The model under review builds one solid part; all positions refer to its coordinate system, in mm. A direction names the side the tool comes from. Round coordinates to 2 decimals unless told otherwise and drop trailing zeros. Loops run counter-clockwise (first coordinate to the right, second up) from the corner with the lowest first, then second, coordinate; pieces in that order, holes last. Notation, with made-up numbers: (14, 82) -> (33, 82) arc R34 cw to (33, 120) -> close; hole circle Ø6 at (34.5, -16.5). An arc over 180 degrees is marked (long way). Use a Markdown table: item, result. Add a question column.
1) Consider section A-A on x = 0. Give the boundary of the cut face in (y, z).
2) For faces 1 (the flat face through (-5, -4, 0)), 2 (the flat face through (5, 4, 0)), 3 (the cylindrical face through (-2.5, -0.1, -15.5)), 4 (the flat face through (-0.1, 2.3, 9)), list the 3-axis set-ups (+Z, -Z, +X, -X, +Y, -Y) from which the entire face can be reached by the end or side of a thin tool; tool diameter is ignored.
3) Consider section B-B on y = 3.25. Give the boundary of the cut face in (x, z).
4) Wall thickness on probe 1 along Z at (x, y) = (3.25, 3.25); probe 2 along Z at (x, y) = (0, 2.25); probe 3 along X at (y, z) = (1.25, -5.5): over which ranges is each line inside the solid? List them lowest first.
5) Consider section C-C on z = -10.5. Give the boundary of the cut face in (x, y).
6) Insertion check: pin 1 (1.3 mm diameter, centred on x = 5, y = 2.5, fed in from -Z); pin 2 (4 mm diameter, centred on y = -3.5, z = -10.5, fed in from +X). Each pin has a flat end and moves straight along its axis. Give the tip position at first contact, or say it passes through.
from build123d import *

# Parameters (mm, degrees)
BOSS_EXTRUDE1_DEPTH      = 9
BOSS_EXTRUDE1_DEPTH_BACK = 15
SKETCH1_W                = 12
SKETCH1_H                = 10
SKETCH3_R                = 8.54
SKETCH3_R_2              = 6
CUT_EXTRUDE_THIN1_DEPTH  = 15
SKETCH5_R                = 2.5
BOSS_EXTRUDE2_DEPTH      = 1
SKETCH6_R                = 1.95
BOSS_EXTRUDE3_DEPTH      = 0.6


with BuildPart() as part:
    # Sketch1 → Boss-Extrude1 (new, two sides: drawn at the far end of the back side and taken through both)
    with BuildSketch(Plane.XY.offset(-BOSS_EXTRUDE1_DEPTH_BACK)):
        Rectangle(SKETCH1_W, SKETCH1_H)
    extrude(amount=BOSS_EXTRUDE1_DEPTH + BOSS_EXTRUDE1_DEPTH_BACK)

    # Sketch3 → Cut-Extrude-Thin1 (cut)
    with BuildSketch(Plane(origin=(0, 0, -15), x_dir=(-1, 0, 0), z_dir=(0, 0, -1))):
        Circle(SKETCH3_R)
        Circle(SKETCH3_R_2, mode=Mode.SUBTRACT)
    extrude(amount=-CUT_EXTRUDE_THIN1_DEPTH, mode=Mode.SUBTRACT)

    # Sketch5 → Boss-Extrude2 (add)
    with BuildSketch(Plane(origin=(0, 0, -15), x_dir=(-1, 0, 0), z_dir=(0, 0, -1))):
        with Locations(Location((0, 0, 0), (0, 0, 180))):
            Circle(SKETCH5_R)
    extrude(amount=BOSS_EXTRUDE2_DEPTH)

    # Sketch6 → Boss-Extrude3 (add)
    with BuildSketch(Plane.XY.offset(9)):
        Circle(SKETCH6_R)
    extrude(amount=BOSS_EXTRUDE3_DEPTH)


solid = part.part
Result set:
| question | item | result |
|---|---|---|
| 1 | outline | (-5, -15) -> (-2.5, -15) -> (-2.5, -16) -> (2.5, -16) -> (2.5, -15) -> (5, -15) -> (5, 9) -> (1.95, 9) -> (1.95, 9.6) -> (-1.95, 9.6) -> (-1.95, 9) -> (-5, 9) -> close |
| 2 | face 1 | -Z, -X, -Y |
| 2 | face 2 | -Z, +X, +Y |
| 2 | face 3 | -Z |
| 2 | face 4 | +Z |
| 3 | outline | (-6, 0) -> (-5.04, 0) -> (-5.04, -15) -> (5.04, -15) -> (5.04, 0) -> (6, 0) -> (6, 9) -> (-6, 9) -> close |
| 4 | probe 1 | -15 to 9 |
| 4 | probe 2 | -16 to 9 |
| 4 | probe 3 | -5.87 to 5.87 |
| 5 | outline | (-3.32, -5) -> (3.32, -5) arc R6 ccw to (3.32, 5) -> (-3.32, 5) arc R6 ccw to start |
| 6 | pin 1 | z = -15 |
| 6 | pin 2 | x = 5.81 |
